Part model, mm, in its own coordinate system. A direction names the side the tool comes from. Give positions to 0.01 mm unless a question says otherwise; leave off trailing zeros. Write each loop counter-clockwise with the first axis right and the second up, starting at its lowest first coordinate (ties: lowest second). Pieces come first, ordered by that corner, then holes. Notation, with made-up numbers: M 34,81.25 L 84,81.25 A12 ccw 84,87.25 Z; hole C -1,55.25 d2. An arc over 180 degrees is marked long. Use CSV: the item, a comma, the result in double quotes. Start each with the question number.
Item 1: Pin check, flat tips, straight feed: pin 1 (1.9 mm diameter, centred on x = 79.5, z = 2, fed in from +Y); pin 2 (3 mm diameter, centred on x = 78, z = 2.5, fed in from -Y); pin 3 (3 mm diameter, centred on x = 5.5, z = 4.5, fed in from +Y). Stop position of each tip, or through.
Item 2: Mould opens along X. For faces 5 (the flat face through (72.5, 20, 3)), 6 (the flat face through (78, 10, 3)), 7 (the flat face through (30, 78, 3)), 8 (the flat face through (71, 20, 3)) say: released by +X, released by -X, zero draft, split by the parting line, or undercut.
Item 3: Cut at A-A (x = 19). List the corners of the cut face in (y, z), then the cut area to 3 significant figures.
Item 4: Cut at C-C (y = 50). List the corners of the cut face in (x, z), then the cut area to 3 significant figures.
Item 5: Drill centre lines: line 1 (Y direction, x = 20.5, z = 4); line 2 (X direction, y = 55.5, z = 4.75); line 3 (Y direction, x = 32.5, z = 0.5). Where is each one in solid material? Low to high. Write a range as [from, to].
Item 6: Which spindle directions (+Z, -Z, +X, -X, +Y, -Y) get a long thin tool onto all of the face, cutting with end or side? Do faces 1 (the flat face through (75, 5, 3)), 2 (the flat face through (5, 75, 3)), 3 (the flat face through (20, 71, 3)), 4 (the flat face through (78, 30, 3)). Say none if no direction does.
Item 7: Cut at B-B (z = 2). List the corners of the cut face in (x, y), then the cut area to 3 significant figures.
Autodesk Inventor part; units mm, degrees
ref_plane "YZ Plane" through (0, 0, 0) normal (1, 0, 0) x (0, 1, 0)
ref_plane "XZ Plane" through (0, 0, 0) normal (0, 1, 0) x (-1, 0, 0)
ref_plane "XY Plane" through (0, 0, 0) normal (0, 0, 1) x (1, 0, 0)
sketch "Sketch1" plane through (0, 0, 0) normal (0, 0, 1) x (1, 0, 0)
  line L0 (0, 75) -> (0, 0)
  line L1 (0, 0) -> (75, 0)
  line L2 (75, 0) -> (75, 40)
  line L3 (75, 40) -> (40, 40)
  line L4 (40, 40) -> (40, 75)
  line L5 (40, 75) -> (0, 75)
  dimension "d0" = 75
  dimension "d2" = 40
extrude "Extrusion1" add sketch "Sketch1" along normal blind 6.477
sketch "Sketch2" plane through (0, 0, 6.477) normal (0, 0, 1) x (1, 0, 0)
  line L0 (75, 0) -> (75, 40)
  line L1 (40, 75) -> (0, 75)
  line L2 (10, 75) -> (30, 75)
  line L3 (30, 75) -> (30, 81.477)
  line L4 (30, 81.477) -> (10, 81.477)
  line L5 (10, 81.477) -> (10, 75)
  line L6 (75, 30) -> (81.477, 30)
  line L7 (81.477, 30) -> (81.477, 10)
  line L8 (81.477, 10) -> (75, 10)
  line L9 (75, 10) -> (75, 30)
  point P0 (75, 20)
  point P1 (20, 75)
  dimension "d5" = 6.477
  dimension "d7" = 20
extrude "Extrusion2" add sketch "Sketch2" against normal up to surface (6.477 mm away)
sketch "Sketch3" plane through (0, 0, 6.477) normal (0, 0, 1) x (1, 0, 0)
  line L0 (81.477, 10) -> (81.477, 30)
  line L1 (75, 30) -> (75, 40)
  line L2 (40, 75) -> (30, 75)
  line L3 (30, 81.477) -> (10, 81.477)
  line L4 (18, 72.5) -> (22, 72.5)
  line L5 (22, 72.5) -> (22, 71)
  line L6 (22, 71) -> (18, 71)
  line L7 (18, 71) -> (18, 72.5)
  line L8 (72.5, 18) -> (71, 18)
  line L9 (71, 18) -> (71, 22)
  line L10 (71, 22) -> (72.5, 22)
  line L11 (72.5, 22) -> (72.5, 18)
  point P0 (72.5, 20)
  point P1 (81.477, 20)
  point P2 (20, 72.5)
  point P3 (20, 81.477)
  dimension "d10" = 2.5
  dimension "d11" = 2.5
  dimension "d12" = 1.5
  dimension "d13" = 4
extrude "Extrusion3" cut sketch "Sketch3" against normal through all
properties part number "OVERHANG SUPPORT"
Worked answers:
1,pin 1,"stops at y = 30"
1,pin 2,"stops at y = 10"
1,pin 3,"stops at y = 75"
2,face 5,"undercut"
2,face 6,"zero draft"
2,face 7,"released by +X"
2,face 8,"undercut"
3,outline,"M 0,0 L 71,0 L 71,6.48 L 0,6.48 Z; M 72.5,0 L 81.48,0 L 81.48,6.48 L 72.5,6.48 Z"
3,area,"518 mm^2"
4,outline,"M 0,0 L 40,0 L 40,6.48 L 0,6.48 Z"
4,area,"259 mm^2"
5,line 1,"y = [0, 71], [72.5, 81.48]"
5,line 2,"x = [0, 40]"
5,line 3,"y = [0, 75]"
6,face 1,"+Z, -Z, +X, -Y"
6,face 2,"+Z, -Z, -X, +Y"
6,face 3,"+Z, -Z"
6,face 4,"+Z, -Z, +X, +Y"
7,outline,"M 0,0 L 75,0 L 75,10 L 81.48,10 L 81.48,30 L 75,30 L 75,40 L 40,40 L 40,75 L 30,75 L 30,81.48 L 10,81.48 L 10,75 L 0,75 Z; hole M 18,71 L 22,71 L 22,72.5 L 18,72.5 Z; hole M 71,18 L 72.5,18 L 72.5,22 L 71,22 Z"
7,area,"4,650 mm^2"
